Can you work these out from the model? Positions are in its coordinate system, mm. Coordinates: 2 decimals unless noted, no trailing zeros. Order: outer loops, then holes, each group sorted by start corner. A loop starts at its lowest first (then second) coordinate and runs counter-clockwise, first axis right, second up. Notation, with made-up numbers: (-28, 60.5) -> (22, 60.5) arc R22 ccw to (22, 77.5) -> close; hole circle Ø10 at (87.5, 11.5). An arc over 180 degrees is marked (long way). Write item = value, one per line.
Autodesk Inventor part; units mm, degrees
ref_plane "YZ Plane" through (0, 0, 0) normal (1, 0, 0) x (0, 1, 0)
ref_plane "XZ Plane" through (0, 0, 0) normal (0, 1, 0) x (-1, 0, 0)
ref_plane "XY Plane" through (0, 0, 0) normal (0, 0, 1) x (1, 0, 0)
sketch "Sketch1" plane through (0, 0, 0) normal (0, 1, 0) x (-1, 0, 0)
  line L0 (0, 329.241) -> (0, -329.241) construction
  line L1 (203.5937, 0) -> (-203.5937, 0) construction
  arc A0 (-441.1, 0) -> (220, -382.3208) centre (0, 0) ccw
  line L2 (-441.1, 0) -> (-441.1, 400)
  line L3 (-441.1, 400) -> (-500, 400)
  line L4 (-500, 400) -> (-500, -500)
  line L5 (-500, -500) -> (220, -500)
  line L6 (220, -500) -> (220, -382.3208)
  dimension "d0" = 500
  dimension "d1" = 400
  dimension "d2" = 500
  dimension "d3" = 441.1
  dimension "d4" = 720
extrude "Extrusion1" add sketch "Sketch1" along normal blind 40
sketch "Sketch3" plane through (0, 0, 0) normal (0, -1, 0) x (1, 0, 0)
  line L0 (339.0044, -382.3208) -> (410, -300.2547)
  line L1 (410, -162.6936) -> (220, -382.3208)
  arc A0 (-220, -382.3208) -> (441.1, 0) centre (0, 0) ccw
  line L2 (500, 400) -> (500, -500)
  line L3 (-595.7823, 565.809) -> (852.8514, 565.809)
  line L4 (852.8514, 565.809) -> (852.8514, -851.0184)
  line L5 (852.8514, -851.0184) -> (-595.7823, -851.0184)
  line L6 (-595.7823, -851.0184) -> (-595.7823, 565.809)
  line L7 (220, -382.3208) -> (339.0044, -382.3208)
  line L8 (410, -162.6936) -> (410, -300.2547)
  dimension "d71" = 90
  dimension "d75" = 90
  dimension "d76" = 290.4068
sketch "Sketch4" plane through (0, 0, 0) normal (0, -1, 0) x (1, 0, 0)
  line L0 (441.1, 400) -> (500, 400) construction
  line L1 (441.1, 0) -> (441.1, 400) construction
  arc A0 (-220, -382.3208) -> (441.1, 0) centre (0, 0) ccw construction
  line L2 (464.3817, -39.9852) -> (0, 0) construction
  line L3 (0, 0) -> (445.1648, -138.1214) construction
  line L4 (423.7332, -194.1633) -> (0, 0) construction
  line L5 (360.2723, -295.7246) -> (0, 0) construction
  line L6 (289.0138, -365.6778) -> (0, 0) construction
  line L7 (389.8771, -255.4312) -> (0, 0) construction
  line L8 (326.5218, -332.615) -> (0, 0) construction
  line L9 (230.9911, -404.8361) -> (0, 0) construction
  line L10 (139.32, -444.7911) -> (0, 0) construction
  line L11 (41.2359, -464.2723) -> (0, 0) construction
  line L12 (464.3817, -39.9852) -> (445.1648, -138.1214) construction
  line L13 (445.1648, -138.1214) -> (423.7332, -194.1633) construction
  line L14 (423.7332, -194.1633) -> (389.8771, -255.4312) construction
  line L15 (389.8771, -255.4312) -> (360.2723, -295.7246) construction
  line L16 (360.2723, -295.7246) -> (326.5218, -332.615) construction
  line L17 (326.5218, -332.615) -> (289.0138, -365.6778) construction
  line L18 (289.0138, -365.6778) -> (230.9911, -404.8361) construction
  line L19 (230.9911, -404.8361) -> (139.32, -444.7911) construction
  line L20 (139.32, -444.7911) -> (41.2359, -464.2723) construction
  line L21 (-58.7462, -462.3831) -> (0, 0) construction
  line L22 (-156.0243, -439.2102) -> (0, 0) construction
  line L23 (-200, -421.0098) -> (0, 0) construction
  line L24 (41.2359, -464.2723) -> (-58.7462, -462.3831) construction
  line L25 (-58.7462, -462.3831) -> (-156.0243, -439.2102) construction
  line L26 (-200, -421.0098) -> (-156.0243, -439.2102) construction
  line L27 (-220, -500) -> (-220, -382.3208) construction
  point P0 (466.1, 360)
  point P1 (466.1, 260)
  point P2 (466.1, 160)
  point P3 (466.1, 60)
  dimension "d50" = 40
  dimension "d51" = 100
  dimension "d52" = 100
  dimension "d53" = 100
  dimension "d54" = 25
  dimension "d55" = 466.1
  dimension "d56" = 100
  dimension "d57" = 100
  dimension "d58" = 60
  dimension "d59" = 70
  dimension "d60" = 50
  dimension "d61" = 70
  dimension "d62" = 100
  dimension "d63" = 20
hole "Hole1" at (-200, 0, -421.0098) at (-156.0243, 0, -439.2102) at (-58.7462, 0, -462.3831) at (41.2359, 0, -464.2723) at (139.32, 0, -444.7911) at (230.9911, 0, -404.8361) at (289.0138, 0, -365.6778) at (326.5218, 0, -332.615) at (360.2723, 0, -295.7246) at (389.8771, 0, -255.4312) at (423.7332, 0, -194.1633) at (445.1648, 0, -138.1214) at (464.3817, 0, -39.9852) at (466.1, 0, 60) at (466.1, 0, 160) at (466.1, 0, 260) at (466.1, 0, 360) direction (0, 1, 0) diameter 5.5 end through all
extrude "Extrusion2" cut sketch "Sketch3" against normal through all
properties part number "boundaryV1"
Item 1: I want a section at B-B, the plane y = 24. Please give me the cut outline in (x, z) (3 decimals), plus the area to 3 significant figures.
A:
outline = (220, -382.321) -> (339.004, -382.321) -> (410, -300.255) -> (410, -162.694) arc R441.1 cw to start; hole circle Ø5.5 at (289.014, -365.678); hole circle Ø5.5 at (326.522, -332.615); hole circle Ø5.5 at (360.272, -295.725); hole circle Ø5.5 at (389.877, -255.431)
area = 13,100 mm2
Item 2: I want a section at D-D, the plane z = -310.5. Please give me the cut outline in (x, y), plus the area to 3 significant figures.
A:
outline = (313.3, 0) -> (401.14, 0) -> (401.14, 40) -> (313.3, 40) -> close
area = 3,510 mm2
Item 3: I want a section at A-A, the plane z = -365.5. Please give me the cut outline in (x, y), plus the area to 3 significant figures.
A:
outline = (246.94, 0) -> (286.27, 0) -> (286.27, 40) -> (246.94, 40) -> close; (291.76, 0) -> (353.56, 0) -> (353.56, 40) -> (291.76, 40) -> close
area = 4,050 mm2
Item 4: If we mould it in two halves opening along Z, with no side actions, what happens to faces 1 (the flat face through (279, 20, -382.321)), 2 (the cylindrical face through (332.23, 19.72, -290.16)), 3 (the cylindrical face through (328.195, 20.28, -330.433))? For each: pulls with the +Z half, pulls with the -Z half, needs draft (parallel to the pull), parting line crosses it, or undercut.
A:
face_1 = pulls with the -Z half
face_2 = pulls with the +Z half
face_3 = undercut
Item 5: I'm going to push flat-ended pins straight in: P1, Ø5, axis at x = 361.5, y = 15, coming from the -Z side; P2, Ø3.5, axis at x = 289.01, z = -365.68, coming from the +Y side; P3, Ø3, axis at y = 14, z = -276.5, coming from the -X side; P4, Ø1.5, axis at x = 364.5, y = 16, coming from the -Z side. Where does each tip first touch, or does it pass through?
A:
P1 = -359.21
P2 = through
P3 = 342.47
P4 = -353.72
Item 6: I want a section at C-C, the plane x = 380. Please give me the cut outline in (y, z), plus the area to 3 significant figures.
A:
outline = (0, -334.93) -> (40, -334.93) -> (40, -223.98) -> (0, -223.98) -> close
area = 4,440 mm2
Item 7: If I drill on probe 1 along X at (y, z) = (35, -366); probe 2 along X at (y, z) = (17.5, -254.5); probe 3 along X at (y, z) = (15, -210), over which ranges is the centre line in solid material (lowest first)?
A:
probe_1 = 246.2 to 286.28, 291.74 to 353.12
probe_2 = 360.28 to 387.29, 392.46 to 410
probe_3 = 387.9 to 410
